from build123d import *

# Parameters (mm, degrees)
F0_W     = 275
F0_H     = 5
F1_DEPTH = 7.5
F2_W     = 275
F2_H     = 11.837108
F3_DEPTH = 5
F4_W     = 42.909291
F4_H     = 10
F5_DEPTH = 5
F6_W     = 275
F6_H     = 11.88611
F7_DEPTH = 5
F8_R     = 1


with BuildPart() as f1:
    # F0 (on Top) → F1 (new body, symmetric)
    with BuildSketch(Plane.XY):
        Rectangle(F0_W, F0_H)
    extrude(amount=F1_DEPTH, both=True)

    # F2 (on face) → F3 (join)
    with BuildSketch(Plane.XY.offset(7.5)):
        with Locations((0, -3.418554)):
            Rectangle(F2_W, F2_H)
    extrude(amount=F3_DEPTH)

    # F4 (on face) → F5 (join)
    with BuildSketch(Plane.XZ.offset(9.337108)):
        with Locations((-116.045355, 7.5)):
            Rectangle(F4_W, F4_H)
        with Locations((116.045355, 7.5)):
            Rectangle(F4_W, F4_H)
    extrude(amount=F5_DEPTH)

    # F6 (on face) → F7 (join)
    with BuildSketch(Plane(origin=(0, 0, -7.5), x_dir=(1, 0, 0), z_dir=(0, 0, -1))):
        with Locations((0, 3.443055)):
            Rectangle(F6_W, F6_H)
    extrude(amount=F7_DEPTH)

    # F8
    f8_edges = [f1.edges().sort_by_distance(p)[0] for p in [
        (0, 2.5, 12.5),
        (0, 2.5, -12.5),
    ]]
    fillet(f8_edges, radius=F8_R)


solid = f1.part
Check sheet for the modelled part. Datum: model origin and axes. Units: mm. A direction names the side the tool comes from. Give positions to 0.01 mm unless a question says otherwise; leave off trailing zeros. Loops run counter-clockwise (first coordinate to the right, second up) from the corner with the lowest first, then second, coordinate; pieces in that order, holes last. Notation, with made-up numbers: M -22,88 L 9,88 A19 ccw 9,120 Z; hole C 33.25,-39 d2. An arc over 180 degrees is marked long. Answer as a JSON object with one key per item and string values. Group by question number.
Q1. Go/stop test with flat-tipped pins: P1, Ø7.5, axis at x = 68, z = -2.5, coming from the -Y side; P2, Ø2.5, axis at x = 31, z = -10, coming from the -Y side; P3, Ø4, axis at x = 45, z = 9, coming from the -Y side. Record where each tip stops, or that it passes through.
Q2. Access from +Z, -Z, +X, -X, +Y, -Y to the whole of each face (thin tool, end or side, straight path). Record for faces 1 (the flat face through (116, -9.337, 5)), 2 (the flat face through (-2, -9.386, -10)), 3 (the flat face through (94.591, -12, 7)).
Q3. Cross-section at B-B on x = 6. Record the cut outline in (y, z), then the cut area to 3 significant figures.
Q4. Cross-section at C-C on z = -3. Record the cut outline in (x, y), then the cut area to 4 significant figures.
Q5. Material ranges on line 1 along Z through (x, y) = (-20, -4); line 2 along X through (y, z) = (-9.5, 4.75); line 3 along Y through (x, z) = (71, 8.5), recorded low to high. Write a range as [from, to].
Q6. Release check for a two-part mould opening along Y. For faces 4 (the flat face through (116, -14.337, 8)), 5 (the flat face through (-2, -6, -7.5)), 6 (the flat face through (-116, -9.337, 5)), 7 (the flat face through (-2, 2.5, 0)) record: released by +Y, released by -Y, zero draft, split by the parting line, or undercut.
Q7. Cross-section at A-A on y = -6.5. Record the cut outline in (x, z).
Q8. Cross-section at D-D on x = 98. Record the cut outline in (y, z).
Evaluation:
{
 "1": {"P1": "stops at y = -2.5", "P2": "stops at y = -9.39", "P3": "stops at y = -9.34"},
 "2": {"face 1": "+X, -X", "face 2": "-Z, +X, -X, -Y", "face 3": "+Z, -Z, -Y"},
 "3": {"outline": "M -9.39,-12.5 L 1.5,-12.5 A1 ccw 2.5,-11.5 L 2.5,11.5 A1 ccw 1.5,12.5 L -9.34,12.5 L -9.34,7.5 L -2.5,7.5 L -2.5,-7.5 L -9.39,-7.5 Z", "area": "193 mm2"},
 "4": {"outline": "M -137.5,-2.5 L 137.5,-2.5 L 137.5,2.5 L -137.5,2.5 Z", "area": "1,375 mm2"},
 "5": {"line 1": "z = [-12.5, -7.5], [7.5, 12.5]", "line 2": "x = [-137.5, -94.59], [94.59, 137.5]", "line 3": "y = [-9.34, 2.5]"},
 "6": {"face 4": "released by -Y", "face 5": "zero draft", "face 6": "undercut", "face 7": "released by +Y"},
 "7": {"outline": "M -137.5,-12.5 L 137.5,-12.5 L 137.5,-7.5 L -137.5,-7.5 Z; M -137.5,7.5 L 137.5,7.5 L 137.5,12.5 L -137.5,12.5 Z"},
 "8": {"outline": "M -14.34,2.5 L -9.34,2.5 L -9.34,7.5 L -2.5,7.5 L -2.5,-7.5 L -9.39,-7.5 L -9.39,-12.5 L 1.5,-12.5 A1 ccw 2.5,-11.5 L 2.5,11.5 A1 ccw 1.5,12.5 L -14.34,12.5 Z"}
}
